Could you check a few things on this model? Use its own coordinates, in mm. A direction names the side the tool comes from. Give positions to 0.01 mm unless a question says otherwise; leave off trailing zeros. Loops run counter-clockwise (first coordinate to the right, second up) from the corner with the lowest first, then second, coordinate; pieces in that order, holes last. Notation, with made-up numbers: M -30,42.25 L -9,42.25 A23 cw -9,67.25 Z; hole C -10,46 d1. An arc over 180 degrees is marked long. Use CSV: the item, a comma, the result in double quotes.
```python
from build123d import *
from OCP.BRepFilletAPI import BRepFilletAPI_MakeChamfer

# Parameters (mm, degrees)
BOSS_EXTRUDE1_DEPTH      = 10.1
BOSS_EXTRUDE1_DEPTH_BACK = 10.1
CUT_EXTRUDE1_REACH       = 44.995
SKETCH2_R                = 2.2
RIB3_REACH               = 43.434
SKETCH3_WALL_W           = 92.969832662
SKETCH3_WALL_H           = 0.8
BOSS_EXTRUDE2_DEPTH      = 2
CHAMFER1_SIZE            = 2
SKETCH5_R                = 6.5
BOSS_EXTRUDE3_DEPTH      = 1.5
CHAMFER2_SIZE            = 3.8
CHAMFER2_SIZE2           = 1.38308689
BOSS_EXTRUDE4_DEPTH      = 3.6
BOSS_EXTRUDE4_DEPTH_BACK = 3.6
FILLET2_R                = 1
SKETCH7_R                = 2.75
SKETCH7_R_2              = 1.35
BOSS_EXTRUDE5_DEPTH      = 3.8
CHAMFER3_SIZE            = 1
CHAMFER3_SIZE2           = 0.363970234


with BuildPart() as part:
    # Sketch1 → Boss-Extrude1 (new, two sides: drawn at the far end of the back side and taken through both)
    with BuildSketch(Plane(origin=(0, 0, 0), x_dir=(0, 0, -1), z_dir=(1, 0, 0)).offset(-BOSS_EXTRUDE1_DEPTH_BACK)):
        Polygon((-8.8, -20.1), (-8.8, 20.1), (-2.3, 20.1), (-2.3, 29.3), (0, 29.3), (0, 20.1), (27.5, 20.1), (27.5, -20.1), (0, -20.1), (0, -29.3), (-2.3, -29.3), (-2.3, -20.1), align=None)
    extrude(amount=BOSS_EXTRUDE1_DEPTH + BOSS_EXTRUDE1_DEPTH_BACK)

    # Sketch2 → Cut-Extrude1 (cut, up to next)
    with BuildSketch(Plane.XY.offset(2.3), mode=Mode.PRIVATE) as cut_extrude1_sk1:
        with Locations((4.525, 24.9)):
            Circle(SKETCH2_R)
    cut_extrude1_tool1 = extrude(cut_extrude1_sk1.sketch, amount=-CUT_EXTRUDE1_REACH, mode=Mode.PRIVATE) & part.part
    # Sketch2 → Cut-Extrude1 (cut, up to next)
    with BuildSketch(Plane.XY.offset(2.3), mode=Mode.PRIVATE) as cut_extrude1_sk2:
        with Locations(Location((-4.525, 24.9, 0), (0, 0, 90))):
            Circle(SKETCH2_R)
    cut_extrude1_tool2 = extrude(cut_extrude1_sk2.sketch, amount=-CUT_EXTRUDE1_REACH, mode=Mode.PRIVATE) & part.part
    # Sketch2 → Cut-Extrude1 (cut, up to next)
    with BuildSketch(Plane.XY.offset(2.3), mode=Mode.PRIVATE) as cut_extrude1_sk3:
        with Locations((-4.525, -24.9)):
            Circle(SKETCH2_R)
    cut_extrude1_tool3 = extrude(cut_extrude1_sk3.sketch, amount=-CUT_EXTRUDE1_REACH, mode=Mode.PRIVATE) & part.part
    # Sketch2 → Cut-Extrude1 (cut, up to next)
    with BuildSketch(Plane.XY.offset(2.3), mode=Mode.PRIVATE) as cut_extrude1_sk4:
        with Locations(Location((4.525, -24.9, 0), (0, 0, 90))):
            Circle(SKETCH2_R)
    cut_extrude1_tool4 = extrude(cut_extrude1_sk4.sketch, amount=-CUT_EXTRUDE1_REACH, mode=Mode.PRIVATE) & part.part
    # Sketch2 → Cut-Extrude1 (cut, up to next)
    with BuildSketch(Plane.XY.offset(2.3), mode=Mode.PRIVATE) as cut_extrude1_sk5:
        with BuildLine():
            Line((-3.65, 29.3), (3.65, 29.3))
            ThreePointArc((3.65, 29.3), (0, 28), (-3.65, 29.3))
        make_face()
    cut_extrude1_tool5 = extrude(cut_extrude1_sk5.sketch, amount=-CUT_EXTRUDE1_REACH, mode=Mode.PRIVATE) & part.part
    # Sketch2 → Cut-Extrude1 (cut, up to next)
    with BuildSketch(Plane.XY.offset(2.3), mode=Mode.PRIVATE) as cut_extrude1_sk6:
        with BuildLine():
            Line((-3.65, -29.3), (3.65, -29.3))
            ThreePointArc((3.65, -29.3), (0, -28), (-3.65, -29.3))
        make_face()
    cut_extrude1_tool6 = extrude(cut_extrude1_sk6.sketch, amount=-CUT_EXTRUDE1_REACH, mode=Mode.PRIVATE) & part.part
    add(cut_extrude1_tool1.solids().sort_by_distance((4.525, 24.9, 2.3))[0], mode=Mode.SUBTRACT)
    add(cut_extrude1_tool2.solids().sort_by_distance((-4.525, 24.9, 2.3))[0], mode=Mode.SUBTRACT)
    add(cut_extrude1_tool3.solids().sort_by_distance((-4.525, -24.9, 2.3))[0], mode=Mode.SUBTRACT)
    add(cut_extrude1_tool4.solids().sort_by_distance((4.525, -24.9, 2.3))[0], mode=Mode.SUBTRACT)
    add(cut_extrude1_tool5.solids().sort_by_distance((0, 28.774631, 2.3))[0], mode=Mode.SUBTRACT)
    add(cut_extrude1_tool6.solids().sort_by_distance((0, -28.774631, 2.3))[0], mode=Mode.SUBTRACT)

    # Sketch3 wall → Rib3 (add, up to next)
    with BuildSketch(Plane(origin=(0, 24.05, 3.2), x_dir=(0, -0.975011472973, 0.222154512829), z_dir=(0, -0.222154512829, -0.975011472973)), mode=Mode.PRIVATE) as rib3_sk1:
        Rectangle(SKETCH3_WALL_W, SKETCH3_WALL_H)
    rib3_tool1 = extrude(rib3_sk1.sketch, amount=RIB3_REACH, mode=Mode.PRIVATE) - part.part
    rib3 = rib3_tool1.solids().sort_by_distance((0, 24.05, 3.2))[0]
    add(rib3)

    # Mirror1: Rib3 across plane
    add(rib3.mirror(Plane.ZX))

    # Sketch4 → Boss-Extrude2 (add)
    with BuildSketch(Plane.XY.offset(8.8)):
        with BuildLine():
            Line((8.9, 5.225065445), (8.9, -16.6))
            Line((8.9, -16.6), (-8.9, -16.6))
            Line((-8.9, -16.6), (-8.9, 5.225065445))
            ThreePointArc((-8.9, 5.225065445), (0, 20.1), (8.9, 5.225065445))
        make_face()
    extrude(amount=BOSS_EXTRUDE2_DEPTH)

    # Chamfer1
    chamfer1_edges = [part.edges().sort_by_distance(p)[0] for p in [
        (0, -16.6, 10.8),
    ]]
    chamfer(chamfer1_edges, length=CHAMFER1_SIZE - 0.0001)  # a hair under: the kernel refuses the full size

    # Sketch5 → Boss-Extrude3 (add)
    with BuildSketch(Plane.XY.offset(10.8)):
        with Locations((0, 10)):
            Circle(SKETCH5_R)
    extrude(amount=BOSS_EXTRUDE3_DEPTH)

    # Chamfer2: one chamfer whose edges measure the first distance from different faces: ONE call of the kernel's chamfer builder (chamfer() names one face for all edges)
    chamfer2_edges_1 = [part.edges().sort_by_distance(p)[0] for p in [
        (-10.1, 0, -27.5),
    ]]
    chamfer2_side_1 = [part.faces().sort_by_distance(p)[0] for p in [
        (-10.1, 0, -9.054071711),
    ]]
    chamfer2_edges_2 = [part.edges().sort_by_distance(p)[0] for p in [
        (0, 20.1, -27.5),
    ]]
    chamfer2_side_2 = [part.faces().sort_by_distance(p)[0] for p in [
        (0, 20.1, -13.75),
    ]]
    chamfer2_edges_3 = [part.edges().sort_by_distance(p)[0] for p in [
        (0, -20.1, -27.5),
    ]]
    chamfer2_side_3 = [part.faces().sort_by_distance(p)[0] for p in [
        (0, -20.1, -13.75),
    ]]
    chamfer2_edges_4 = [part.edges().sort_by_distance(p)[0] for p in [
        (10.1, 0, -27.5),
    ]]
    chamfer2_side_4 = [part.faces().sort_by_distance(p)[0] for p in [
        (10.1, 0, -9.054071711),
    ]]
    chamfer2 = BRepFilletAPI_MakeChamfer(part.part.solid().wrapped)
    for e in chamfer2_edges_1:
        chamfer2.Add(CHAMFER2_SIZE, CHAMFER2_SIZE2, e.wrapped, chamfer2_side_1[0].wrapped)  # the first distance lies on this face
    for e in chamfer2_edges_2:
        chamfer2.Add(CHAMFER2_SIZE, CHAMFER2_SIZE2, e.wrapped, chamfer2_side_2[0].wrapped)  # the first distance lies on this face
    for e in chamfer2_edges_3:
        chamfer2.Add(CHAMFER2_SIZE, CHAMFER2_SIZE2, e.wrapped, chamfer2_side_3[0].wrapped)  # the first distance lies on this face
    for e in chamfer2_edges_4:
        chamfer2.Add(CHAMFER2_SIZE, CHAMFER2_SIZE2, e.wrapped, chamfer2_side_4[0].wrapped)  # the first distance lies on this face
    add(Compound.cast(chamfer2.Shape()), mode=Mode.REPLACE)

    # Sketch6 → Boss-Extrude4 (add, two sides: drawn at the far end of the back side and taken through both)
    with BuildSketch(Plane(origin=(0, 0, 0), x_dir=(0, 0, -1), z_dir=(1, 0, 0)).offset(-BOSS_EXTRUDE4_DEPTH_BACK)):
        Polygon((25.65, 18.71691311), (20.95, 18.71691311), (20.95, 21.1), (21.95, 21.1), (21.95, 24.6), (24.65, 24.6), (24.65, 21.110599186), (25.65, 21.110599186), align=None)
    extrude(amount=BOSS_EXTRUDE4_DEPTH + BOSS_EXTRUDE4_DEPTH_BACK)

    # Fillet2
    fillet2_edges = [part.edges().sort_by_distance(p)[0] for p in [
        (-3.6, 22.85, -21.95),
        (-3.6, 22.855299593, -24.65),
        (3.6, 22.855299593, -24.65),
        (3.6, 22.85, -21.95),
    ]]
    fillet(fillet2_edges, radius=FILLET2_R)

    # Sketch7 → Boss-Extrude5 (add)
    with BuildSketch(Plane.XY.offset(12.3)):
        with Locations(Location((0, 10, 0), (0, 0, 180))):
            Circle(SKETCH7_R)
        with Locations(Location((0, 10, 0), (0, 0, 180))):
            Circle(SKETCH7_R_2, mode=Mode.SUBTRACT)
    extrude(amount=BOSS_EXTRUDE5_DEPTH)

    # Chamfer3
    chamfer3_edges = [part.edges().sort_by_distance(p)[0] for p in [
        (2.75, 10, 16.1),
    ]]
    chamfer3_side = [part.faces().sort_by_distance(p)[0] for p in [
        (2.75, 10, 14.2),
    ]]
    chamfer(chamfer3_edges, length=CHAMFER3_SIZE, length2=CHAMFER3_SIZE2, reference=chamfer3_side[0])


solid = part.part
```
1. If we mould it in two halves opening along Z, with no side actions, what happens to faces 1 (the face through (0, 24.6, -23)), 2 (the face through (-0.1, 21.1, -21.5)), 3 (the face through (-0.006, 24.105, 3.187))? For each: +Z half, -Z half, draft (parallel to the pull), parting line (faces both ways), or undercut.
Outcome:
face 1,"draft"
face 2,"undercut"
face 3,"+Z half"
2. I want a section at C-C, the plane z = -9. List the corners of the cut face in (x, y) for me.
Outcome:
outline,"M -10.1,-20.1 L 10.1,-20.1 L 10.1,20.1 L -10.1,20.1 Z"
3. I want a section at B-B, the plane y = -24.9. List the corners of the cut face in (x, z) for me (3 decimals), then the cut area to 3 significant figures.
Outcome:
outline,"M -10.1,0 L -6.725,0 L -6.725,2.3 L -10.1,2.3 Z; M -2.325,0 L 2.325,0 L 2.325,2.3 L 0.4,2.3 L 0.4,3.006 L -0.4,3.006 L -0.4,2.3 L -2.325,2.3 Z; M 6.725,0 L 10.1,0 L 10.1,2.3 L 6.725,2.3 Z"
area,"26.8 mm2"
4. I'm going to push flat-ended pins straight in: pin 1 Ø8 at (x, z) = (-0.5, -14.5) entering from -Y; pin 2 Ø0.9 at (x, y) = (-1, 20) entering from -Z; pin 3 Ø1.6 at (y, z) = (-1.5, 10) entering from -X. Where does each tip first touch, or does it pass through?
Outcome:
pin 1,"y = -20.1"
pin 2,"z = -25.65"
pin 3,"x = -8.9"
5. Please list where these lines run through material, in increasing order: line 1 (Y direction, x = 0, z = 15); line 2 (Y direction, x = -6, z = 2); line 3 (Z direction, x = 0, y = 9).
Outcome:
line 1,"7.25 to 8.65, 11.35 to 12.75"
line 2,"-29.3 to -26.53, -23.27 to 23.27, 26.53 to 29.3"
line 3,"-27.5 to 12.3"
6. I want a section at A-A, the plane y = -7.5. List the corners of the cut face in (x, z) for me, then the cut area to 3 significant figures.
Outcome:
outline,"M -10.1,-23.7 L -8.72,-27.5 L 8.72,-27.5 L 10.1,-23.7 L 10.1,8.8 L 8.9,8.8 L 8.9,10.8 L -8.9,10.8 L -8.9,8.8 L -10.1,8.8 Z"
area,"764 mm2"
7. Which directions (+Z, -Z, +X, -X, +Y, -Y) give clear straight access to the entire face, cutting with the end or side of a thin tool? Please do faces 4 (the face through (-6, -23, 2.3)), 5 (the face through (8, 18, 8.8)), 6 (the face through (0, -17, 8.8)).
Outcome:
face 4,"+Z, -X, -Y"
face 5,"+Z, +X, +Y"
face 6,"+Z, -Y"
